Input: part model. Units: mm. Frame: model coordinates. Face numbers are marked on the shaded views. A direction names the side the tool comes from. Round coordinates to 2 decimals unless told otherwise and drop trailing zeros. Loops run counter-clockwise (first coordinate to the right, second up) from the corner with the lowest first, then second, coordinate; pieces in that order, holes last.
(1) First-contact query: pin 1 Ø12 at (x, z) = (-67.5, -43) entering from -Y (3 decimals); pin 2 Ø8.5 at (x, z) = (-94.04, 40.88) entering from -Y. Flat tips, straight axial feed; report the tip coordinate or a pass-through.
(2) Line query: line 1 (X direction, y = -44, z = 47); line 2 (Y direction, x = -21.5, z = -20.5) (3 decimals). Output: solid intervals per line, ascending.
(3) Draft query along X for the marked faces 3, 4 and 5. Return one class per face: released by +X, released by -X, zero draft, split by the parting line, or undercut.
(4) Cut plane C-C, the plane x = 20. Output: boundary loops of the cut face in (y, z) (3 decimals).
(5) Cut plane B-B, the plane z = -32.5. Output: boundary loops of the cut face in (x, y) (3 decimals).
(6) Access query for the marked faces 1 and 2. Directions: +Z, -Z, +X, -X, +Y, -Y. A direction counts if a zero-diameter tool reaches every point of the face in a straight line with its end or side. Return the directions, or none.
(7) Cut plane A-A, the plane y = -13. Output: boundary loops of the cut face in (x, z), and give its area (3 significant figures).
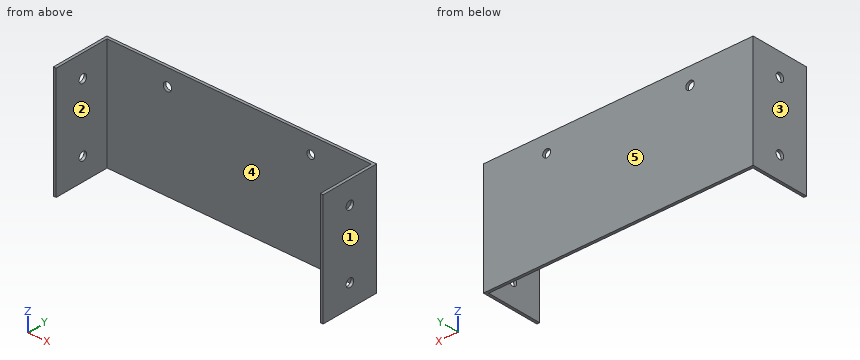
from build123d import *

# Parameters (mm, degrees)
F0_W     = 304.8
F0_H     = 127
F1_DEPTH = 3.175
F2_W     = 3.175
F2_H     = 127
F3_DEPTH = 63.5
F4_R     = 4.7625
F4_R_2   = 4.47244
F5_DEPTH = 25.4
F6_R     = 4.7625
F7_DEPTH = 304.8


with BuildPart() as f1:
    # F0 (on Front) → F1 (new body)
    with BuildSketch(Plane.XZ):
        with Locations((-13.010172, -3.574955)):
            Rectangle(F0_W, F0_H)
    extrude(amount=F1_DEPTH)

    # F2 (on face) → F3 (join)
    with BuildSketch(Plane.XZ.offset(3.175)):
        with Locations((-163.822672, -3.574955)):
            Rectangle(F2_W, F2_H)
        with Locations((137.802328, -3.574955)):
            Rectangle(F2_W, F2_H)
    extrude(amount=F3_DEPTH)

    # F4 (on face) → F5 (cut)
    with BuildSketch(Plane.XZ.offset(3.175)):
        with Locations((-94.036172, 40.875045)):
            Circle(F4_R)
        with Locations((67.888828, 40.875045)):
            Circle(F4_R_2)
    extrude(amount=-F5_DEPTH, mode=Mode.SUBTRACT)

    # F6 (on face) → F7 (cut)
    with BuildSketch(Plane.YZ.offset(139.389828)):
        with Locations((-33.3375, 34.525045)):
            Circle(F6_R)
        with Locations((-33.3375, -41.674955)):
            Circle(F6_R)
    extrude(amount=-F7_DEPTH, mode=Mode.SUBTRACT)


solid = f1.part
Reported:
1. pin 1: stops at y = -3.175
1. pin 2: passes through
2. line 1: x = -165.41 to -162.24, 136.21 to 139.39
2. line 2: y = -3.175 to 0
3. face 3: released by -X
3. face 4: undercut
3. face 5: zero draft
4. outline: (-3.175, -67.075) - (0, -67.075) - (0, 59.925) - (-3.175, 59.925) - close
5. outline: (-165.41, -66.675) - (-162.235, -66.675) - (-162.235, -3.175) - (136.215, -3.175) - (136.215, -66.675) - (139.39, -66.675) - (139.39, 0) - (-165.41, 0) - close
6. face 1: +Z, -Z, +X, +Y, -Y
6. face 2: +Z, -Z, -Y
7. outline: (-165.41, -67.07) - (-162.24, -67.07) - (-162.24, 59.93) - (-165.41, 59.93) - close; (136.21, -67.07) - (139.39, -67.07) - (139.39, 59.93) - (136.21, 59.93) - close
7. area: 806 mm2
